```python
from build123d import *

# Parameters (mm, degrees)
BOSS_EXTRUDE1_DEPTH           = 4
BOSS_EXTRUDE1_DRAFT           = 1
SHELL1_T                      = -0.5
BOSS_EXTRUDE2_DEPTH           = 5.5
BOSS_EXTRUDE2_DRAFT           = 1.5
BOSS_EXTRUDE2_PROFILE_2_DEPTH = 5.5
BOSS_EXTRUDE2_PROFILE_2_DRAFT = 1.5
BOSS_EXTRUDE2_PROFILE_3_DEPTH = 5.5
BOSS_EXTRUDE2_PROFILE_3_DRAFT = 1.5
BOSS_EXTRUDE2_PROFILE_4_DEPTH = 5.5
BOSS_EXTRUDE2_PROFILE_4_DRAFT = 1.5


with BuildPart() as part:
    # Sketch1 → Boss-Extrude1 (with draft: the straight prism first)
    with BuildSketch(Plane(origin=(0, 0, 0), x_dir=(1, 0, 0), z_dir=(0, 1, 0))):
        with BuildLine():
            Line((-7.5, -4), (7.5, -4))
            ThreePointArc((7.5, -4), (8.207106781, -3.707106781), (8.5, -3))
            Line((8.5, -3), (8.5, 3))
            ThreePointArc((8.5, 3), (8.207106781, 3.707106781), (7.5, 4))
            Line((7.5, 4), (-7.5, 4))
            ThreePointArc((-7.5, 4), (-8.207106781, 3.707106781), (-8.5, 3))
            Line((-8.5, 3), (-8.5, -3))
            ThreePointArc((-8.5, -3), (-8.207106781, -3.707106781), (-7.5, -4))
        make_face()
    extrude(amount=-BOSS_EXTRUDE1_DEPTH)
    # Boss-Extrude1: the draft: its side faces are tilted about the plane it starts from
    boss_extrude1_sides = [part.faces().sort_by_distance(p)[0] for p in [
        (0, -2, 4),
        (8.207106781, -2, 3.707106781),
        (8.5, -2, 0),
        (8.207106781, -2, -3.707106781),
        (0, -2, -4),
        (-8.207106781, -2, -3.707106781),
        (-8.5, -2, 0),
        (-8.207106781, -2, 3.707106781),
    ]]
    draft(boss_extrude1_sides, Plane(origin=(0, 0, 0), x_dir=(1, 0, 0), z_dir=(0, 1, 0)), BOSS_EXTRUDE1_DRAFT)

    # Shell1
    shell1_openings = [part.faces().sort_by_distance(p)[0] for p in [
        (0, -4, 0),
    ]]
    offset(amount=SHELL1_T, openings=shell1_openings, kind=Kind.INTERSECTION)


with BuildPart() as boss_extrude2_tool:
    # Sketch2 → Boss-Extrude2 (with draft: the straight prism first)
    with BuildSketch(Plane.XZ.offset(0.5)):
        with BuildLine():
            ThreePointArc((-0.6, 2.93078798), (-2.115362638, 2.115362638), (-2.93078798, 0.6))
            Line((-2.93078798, 0.6), (-0.6, 0.6))
            Line((-0.6, 0.6), (-0.6, 2.93078798))
        make_face()
    extrude(amount=BOSS_EXTRUDE2_DEPTH)
    # Boss-Extrude2: the draft: its side faces are tilted about the plane it starts from
    boss_extrude2_sides = [boss_extrude2_tool.faces().sort_by_distance(p)[0] for p in [
        (-2.115362638, -3.25, 2.115362638),
        (-1.76539399, -3.25, 0.6),
        (-0.6, -3.25, 1.76539399),
    ]]
    draft(boss_extrude2_sides, Plane.XZ.offset(0.5), BOSS_EXTRUDE2_DRAFT)


with BuildPart() as part_1:
    add(part.part)

    # Boss-Extrude2: add boss_extrude2_tool
    add(boss_extrude2_tool.part)


with BuildPart() as boss_extrude2_profile_2_tool:
    # Sketch2 → Boss-Extrude2 profile 2 (with draft: the straight prism first)
    with BuildSketch(Plane.XZ.offset(0.5)):
        with BuildLine():
            ThreePointArc((-2.93078798, -0.6), (-2.115362638, -2.115362638), (-0.6, -2.93078798))
            Line((-0.6, -2.93078798), (-0.6, -0.6))
            Line((-0.6, -0.6), (-2.93078798, -0.6))
        make_face()
    extrude(amount=BOSS_EXTRUDE2_PROFILE_2_DEPTH)
    # Boss-Extrude2 profile 2: the draft: its side faces are tilted about the plane it starts from
    boss_extrude2_profile_2_sides = [boss_extrude2_profile_2_tool.faces().sort_by_distance(p)[0] for p in [
        (-2.115362638, -3.25, -2.115362638),
        (-0.6, -3.25, -1.76539399),
        (-1.76539399, -3.25, -0.6),
    ]]
    draft(boss_extrude2_profile_2_sides, Plane.XZ.offset(0.5), BOSS_EXTRUDE2_PROFILE_2_DRAFT)


with BuildPart() as part_2:
    add(part_1.part)

    # Boss-Extrude2 profile 2: add boss_extrude2_profile_2_tool
    add(boss_extrude2_profile_2_tool.part)


with BuildPart() as boss_extrude2_profile_3_tool:
    # Sketch2 → Boss-Extrude2 profile 3 (with draft: the straight prism first)
    with BuildSketch(Plane.XZ.offset(0.5)):
        with BuildLine():
            Line((0.6, 2.93078798), (0.6, 0.6))
            Line((0.6, 0.6), (2.93078798, 0.6))
            ThreePointArc((2.93078798, 0.6), (2.115362638, 2.115362638), (0.6, 2.93078798))
        make_face()
    extrude(amount=BOSS_EXTRUDE2_PROFILE_3_DEPTH)
    # Boss-Extrude2 profile 3: the draft: its side faces are tilted about the plane it starts from
    boss_extrude2_profile_3_sides = [boss_extrude2_profile_3_tool.faces().sort_by_distance(p)[0] for p in [
        (2.115362638, -3.25, 2.115362638),
        (0.6, -3.25, 1.76539399),
        (1.76539399, -3.25, 0.6),
    ]]
    draft(boss_extrude2_profile_3_sides, Plane.XZ.offset(0.5), BOSS_EXTRUDE2_PROFILE_3_DRAFT)


with BuildPart() as part_3:
    add(part_2.part)

    # Boss-Extrude2 profile 3: add boss_extrude2_profile_3_tool
    add(boss_extrude2_profile_3_tool.part)


with BuildPart() as boss_extrude2_profile_4_tool:
    # Sketch2 → Boss-Extrude2 profile 4 (with draft: the straight prism first)
    with BuildSketch(Plane.XZ.offset(0.5)):
        with BuildLine():
            Line((0.6, -0.6), (0.6, -2.93078798))
            ThreePointArc((0.6, -2.93078798), (2.115362638, -2.115362638), (2.93078798, -0.6))
            Line((2.93078798, -0.6), (0.6, -0.6))
        make_face()
    extrude(amount=BOSS_EXTRUDE2_PROFILE_4_DEPTH)
    # Boss-Extrude2 profile 4: the draft: its side faces are tilted about the plane it starts from
    boss_extrude2_profile_4_sides = [boss_extrude2_profile_4_tool.faces().sort_by_distance(p)[0] for p in [
        (1.76539399, -3.25, -0.6),
        (0.6, -3.25, -1.76539399),
        (2.115362638, -3.25, -2.115362638),
    ]]
    draft(boss_extrude2_profile_4_sides, Plane.XZ.offset(0.5), BOSS_EXTRUDE2_PROFILE_4_DRAFT)


with BuildPart() as part_4:
    add(part_3.part)

    # Boss-Extrude2 profile 4: add boss_extrude2_profile_4_tool
    add(boss_extrude2_profile_4_tool.part)


solid = part_4.part
```
Geometry check sheet. Reference: the model listing, model coordinates, mm. A direction names the side the tool comes from. Give positions to 0.01 mm unless a question says otherwise; leave off trailing zeros. Write each loop counter-clockwise with the first axis right and the second up, starting at its lowest first coordinate (ties: lowest second). Pieces come first, ordered by that corner, then holes.
1) Section check D-D, the plane x = 0.25. Record the boundary of the cut face in (y, z).
2) Material ranges on L1, parallel to X at y = -2.5, z = -2.5; L2, parallel to Z at x = 2, y = -3.5; L3, parallel to X at y = -2.25, z = -2, recorded low to high.
3) Release check for a two-part mould opening along X. For faces 4 (the conical face through (2.08, -3.21, 2.05)), 5 (the conical face through (-8.22, -1.97, -3.74)), 6 (the conical face through (8.24, -1.97, -3.72)), 7 (the flat face through (1.5, -6, 1.5)) record: pulls with the +X half, pulls with the -X half, needs draft (parallel to the pull), parting line crosses it, or undercut.
4) Section check B-B, the plane z = 0. Record the boundary of the cut face in (x, y).
5) Section check A-A, the plane y = -2.5. Record the boundary of the cut face in (x, z), and give its area (3 significant figures).
6) Section check C-C, the plane y = -0.75. Record the boundary of the cut face in (x, z).
7) Gauge pin test, flat ends, axial feed: pin 1 (1 mm diameter, centred on x = -5.5, y = -1, fed in from +Z); pin 2 (1 mm diameter, centred on x = 1.5, z = -3, fed in from +Y); pin 3 (1 mm diameter, centred on x = -2.5, y = -2.5, fed in from -Z); pin 4 (2 mm diameter, centred on x = -6.5, z = -3, fed in from -Y). Record the tip position at first contact, or that the pin passes through.
8) Access from +Z, -Z, +X, -X, +Y, -Y to the whole of each face (thin tool, end or side, straight path). Record for faces 1 (the conical face through (-8.24, -1.97, 3.72)), 2 (the conical face through (-2.08, -3.21, -2.05)), 3 (the flat face through (-1.5, -6, 1.5)).
Computed:
1. outline: (-4, -4.07) - (0, -4) - (0, 4) - (-4, 4.07) - (-4, 3.57) - (-0.5, 3.51) - (-0.5, -3.51) - (-4, -3.57) - close
2. L1: x = -8.54 to -8.04, -1.55 to -0.65, 0.65 to 1.55, 8.04 to 8.54
2. L2: z = -4.06 to -3.56, -2.12 to -0.68, 0.68 to 2.12, 3.56 to 4.06
2. L3: x = -8.54 to -8.04, -2.16 to -0.65, 0.65 to 2.16, 8.04 to 8.54
3. face 4: undercut
3. face 5: pulls with the -X half
3. face 6: pulls with the +X half
3. face 7: needs draft
4. outline: (-8.57, -4) - (-8.07, -4) - (-8.01, -0.5) - (8.01, -0.5) - (8.07, -4) - (8.57, -4) - (8.5, 0) - (-8.5, 0) - close
5. outline: (-8.54, -3) arc R1.04 ccw to (-7.5, -4.04) - (7.5, -4.04) arc R1.04 ccw to (8.54, -3) - (8.54, 3) arc R1.04 ccw to (7.5, 4.04) - (-7.5, 4.04) arc R1.04 ccw to (-8.54, 3) - close; (-2.87, -0.65) arc R2.94 ccw to (-0.65, -2.87) - (-0.65, -0.65) - close; (-2.87, 0.65) - (-0.65, 0.65) - (-0.65, 2.87) arc R2.94 ccw to start; (0.65, -2.87) arc R2.94 ccw to (2.87, -0.65) - (0.65, -0.65) - close; (0.65, 0.65) - (2.87, 0.65) arc R2.94 ccw to (0.65, 2.87) - close; hole (-8.04, -3) arc R0.54 ccw to (-7.5, -3.54) - (7.5, -3.54) arc R0.54 ccw to (8.04, -3) - (8.04, 3) arc R0.54 ccw to (7.5, 3.54) - (-7.5, 3.54) arc R0.54 ccw to (-8.04, 3) - close
5. area: 37.1 mm2
6. outline: (-8.51, -3) arc R1.01 ccw to (-7.5, -4.01) - (7.5, -4.01) arc R1.01 ccw to (8.51, -3) - (8.51, 3) arc R1.01 ccw to (7.5, 4.01) - (-7.5, 4.01) arc R1.01 ccw to (-8.51, 3) - close; (-2.92, -0.61) arc R2.99 ccw to (-0.61, -2.92) - (-0.61, -0.61) - close; (-2.92, 0.61) - (-0.61, 0.61) - (-0.61, 2.92) arc R2.99 ccw to start; (0.61, -2.92) arc R2.99 ccw to (2.92, -0.61) - (0.61, -0.61) - close; (0.61, 0.61) - (2.92, 0.61) arc R2.99 ccw to (0.61, 2.92) - close; hole (-8.01, -3) arc R0.51 ccw to (-7.5, -3.51) - (7.5, -3.51) arc R0.51 ccw to (8.01, -3) - (8.01, 3) arc R0.51 ccw to (7.5, 3.51) - (-7.5, 3.51) arc R0.51 ccw to (-8.01, 3) - close
7. pin 1: stops at z = 4.03
7. pin 2: stops at y = 0
7. pin 3: stops at z = -4.05
7. pin 4: stops at y = -4
8. face 1: +Z, -X, +Y
8. face 2: -Y
8. face 3: +Z, -Z, +X, -X, -Y
